from build123d import *

# Parameters (mm, degrees)
SKETCH1_W           = 22
SKETCH1_H           = 20
BOSS_EXTRUDE1_DEPTH = 22
SKETCH2_W           = 12
SKETCH2_H           = 12
CUT_EXTRUDE1_DEPTH  = 15
SKETCH3_W           = 22
SKETCH3_H           = 5
BOSS_EXTRUDE2_DEPTH = 2
LPATTERN1_COUNT     = 6
LPATTERN1_PITCH     = 24
SKETCH4_W           = 22
SKETCH4_H           = 15
BOSS_EXTRUDE3_DEPTH = 2
SKETCH5_W           = 22
SKETCH5_H           = 20
BOSS_EXTRUDE4_DEPTH = 2
SKETCH6_W           = 132
SKETCH6_H           = 2
CUT_EXTRUDE2_DEPTH  = 2
SKETCH7_W           = 146
SKETCH7_H           = 22
BOSS_EXTRUDE5_DEPTH = 6


with BuildPart() as part:
    # Sketch1 → Boss-Extrude1 (new body)
    with BuildSketch(Plane.XY):
        with Locations((11, 10)):
            Rectangle(SKETCH1_W, SKETCH1_H)
    extrude(amount=BOSS_EXTRUDE1_DEPTH)

    # Sketch2 → Cut-Extrude1 (cut)
    with BuildSketch(Plane.XZ):
        with Locations((11, 11)):
            Rectangle(SKETCH2_W, SKETCH2_H)
    extrude(amount=-CUT_EXTRUDE1_DEPTH, mode=Mode.SUBTRACT)

    # Sketch3 → Boss-Extrude2 (add)
    with BuildSketch(Plane(origin=(22, 0, 0), x_dir=(0, 0, -1), z_dir=(1, 0, 0))):
        with Locations((-11, 2.5)):
            Rectangle(SKETCH3_W, SKETCH3_H)
    extrude(amount=BOSS_EXTRUDE2_DEPTH)


with BuildPart() as lpattern1_1:
    # LPattern1: pattern copy
    add(part.part.moved(Location(Vector(1, 0, 0) * (1 * LPATTERN1_PITCH))))


with BuildPart() as lpattern1_2:
    # LPattern1: pattern copy
    add(part.part.moved(Location(Vector(1, 0, 0) * (2 * LPATTERN1_PITCH))))


with BuildPart() as lpattern1_3:
    # LPattern1: pattern copy
    add(part.part.moved(Location(Vector(1, 0, 0) * (3 * LPATTERN1_PITCH))))


with BuildPart() as lpattern1_4:
    # LPattern1: pattern copy
    add(part.part.moved(Location(Vector(1, 0, 0) * (4 * LPATTERN1_PITCH))))


with BuildPart() as lpattern1_5:
    # LPattern1: pattern copy
    add(part.part.moved(Location(Vector(1, 0, 0) * (5 * LPATTERN1_PITCH))))


with BuildPart() as lpattern1_2_1:
    add(lpattern1_2.part)

    # Combine1: union LPattern1_3, LPattern1_4, LPattern1_5, LPattern1_1, part
    add(lpattern1_3.part)
    add(lpattern1_4.part)
    add(lpattern1_5.part)
    add(lpattern1_1.part)
    add(part.part)

    # Sketch4 → Boss-Extrude3 (add)
    with BuildSketch(Plane(origin=(142, 0, 0), x_dir=(0, 0, -1), z_dir=(1, 0, 0))):
        with Locations((-11, 12.5)):
            Rectangle(SKETCH4_W, SKETCH4_H)
    extrude(amount=BOSS_EXTRUDE3_DEPTH)

    # Sketch5 → Boss-Extrude4 (add)
    with BuildSketch(Plane.ZY):
        with Locations((11, 10)):
            Rectangle(SKETCH5_W, SKETCH5_H)
    extrude(amount=BOSS_EXTRUDE4_DEPTH)

    # Sketch6 → Cut-Extrude2 (cut)
    with BuildSketch(Plane(origin=(0, 0, 0), x_dir=(-1, 0, 0), z_dir=(0, -1, 0))):
        with Locations((-71, -11)):
            Rectangle(SKETCH6_W, SKETCH6_H)
    extrude(amount=-CUT_EXTRUDE2_DEPTH, mode=Mode.SUBTRACT)

    # Sketch7 → Boss-Extrude5 (add)
    with BuildSketch(Plane(origin=(0, 0, 0), x_dir=(-1, 0, 0), z_dir=(0, -1, 0))):
        with Locations((-71, -11)):
            Rectangle(SKETCH7_W, SKETCH7_H)
    extrude(amount=BOSS_EXTRUDE5_DEPTH)


solid = lpattern1_2_1.part
Design review of the part built by this model. Coordinates are the model's own, in mm. A direction names the side the tool comes from. Give positions to 0.01 mm unless a question says otherwise; leave off trailing zeros. Loops run counter-clockwise (first coordinate to the right, second up) from the corner with the lowest first, then second, coordinate; pieces in that order, holes last. Notation, with made-up numbers: (24.5, 73.25) -> (73.5, 73.25) arc R33 ccw to (73.5, 110.25) -> close; hole circle Ø3 at (-38.75, 18). An arc over 180 degrees is marked (long way). One line per question, with ' | ' between items. Start each with the question number.
(1) We need section B-B (x = 107.5). State the section outline as (y, z) points, and give its area (3 significant figures).
(2) Draft analysis for pull direction X (two halves, no side actions). For faces 4 (the face through (5, 7, 11)), 5 (the face through (83, 20, 11)), 6 (the face through (-2, 7, 11)), state which applies: +X half, -X half, draft (parallel to the pull), parting line (faces both ways), or undercut.
(3) For line 1 (Y direction, x = 31, z = 8.75); line 2 (Z direction, x = 109, y = 3.25); line 3 (Y direction, x = 25, z = 10.75), list the stretches that pass through material, from the lowest coordinate up.
(4) We need section A-A (y = 17). State the section outline as (x, z) points.
(5) For faces 1 (the face through (41, 7, 11)), 2 (the face through (46, 12, 11)), 3 (the face through (132, 20, 11)), list the 3-axis set-ups (+Z, -Z, +X, -X, +Y, -Y) from which the entire face can be reached by the end or side of a thin tool; tool diameter is ignored.
(6) We need section C-C (z = 19.5). State the section outline as (x, y) points.
(7) We need section D-D (y = 3.75). State the section outline as (x, z) points.
The answers:
1) outline: (-6, 0) -> (20, 0) -> (20, 22) -> (-6, 22) -> close; hole (0, 5) -> (15, 5) -> (15, 17) -> (0, 17) -> close | area: 392 mm^2
2) face 4: undercut | face 5: draft | face 6: -X half
3) line 1: y = -6 to 0, 15 to 20 | line 2: z = 0 to 5, 17 to 22 | line 3: y = -6 to 0, 2 to 20
4) outline: (-2, 0) -> (22, 0) -> (22, 22) -> (-2, 22) -> close; (24, 0) -> (46, 0) -> (46, 22) -> (24, 22) -> close; (48, 0) -> (70, 0) -> (70, 22) -> (48, 22) -> close; (72, 0) -> (94, 0) -> (94, 22) -> (72, 22) -> close; (96, 0) -> (118, 0) -> (118, 22) -> (96, 22) -> close; (120, 0) -> (144, 0) -> (144, 22) -> (120, 22) -> close
5) face 1: none | face 2: +Z, -Z, +Y | face 3: +Z, -Z, +X, -X, +Y
6) outline: (-2, -6) -> (144, -6) -> (144, 20) -> (120, 20) -> (120, 5) -> (118, 5) -> (118, 20) -> (96, 20) -> (96, 5) -> (94, 5) -> (94, 20) -> (72, 20) -> (72, 5) -> (70, 5) -> (70, 20) -> (48, 20) -> (48, 5) -> (46, 5) -> (46, 20) -> (24, 20) -> (24, 5) -> (22, 5) -> (22, 20) -> (-2, 20) -> close
7) outline: (-2, 0) -> (144, 0) -> (144, 22) -> (-2, 22) -> close; hole (5, 5) -> (17, 5) -> (17, 17) -> (5, 17) -> close; hole (29, 5) -> (41, 5) -> (41, 17) -> (29, 17) -> close; hole (53, 5) -> (65, 5) -> (65, 17) -> (53, 17) -> close; hole (77, 5) -> (89, 5) -> (89, 17) -> (77, 17) -> close; hole (101, 5) -> (113, 5) -> (113, 17) -> (101, 17) -> close; hole (125, 5) -> (137, 5) -> (137, 17) -> (125, 17) -> close
